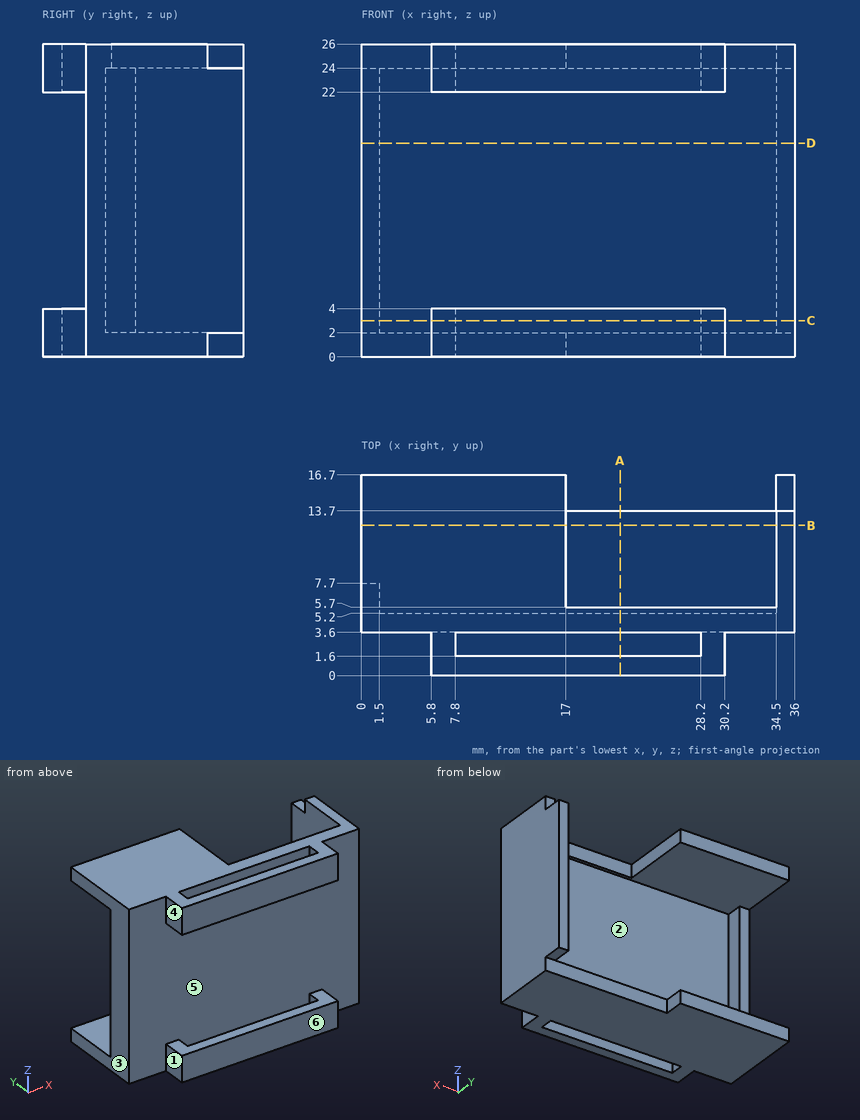
Can you work these out from the drawing? Everything is in mm from the part's minimum corner. A direction names the side the tool comes from. Give positions to 0.01 mm unless a question says otherwise; leave off trailing zeros. Write each loop counter-clockwise with the first axis right and the second up, starting at its lowest first coordinate (ties: lowest second). Pieces come first, ordered by that corner, then holes. Notation, with made-up numbers: (-4.5, 39) -> (40.5, 39) arc R30 ccw to (40.5, 68) -> close; hole circle Ø8 at (32, 30). An arc over 180 degrees is marked (long way). Write each question's results on one line, items separated by ' | '.
Item 1: If I drill on L1, parallel to Z at x = 15, y = 1; L2, parallel to Z at x = 28.5, y = 5.25; L3, parallel to X at y = 6.25, z = 3.5, over which ranges is the centre line in solid material (lowest first)?
Output:
L1: z = 0 to 4, 22 to 26 | L2: z = 0 to 2, 24 to 26 | L3: x = 0 to 1.5, 34.5 to 36
Item 2: Suppose I cut it at D-D on z = 17.75. Write out the boundary of the cut face in (x, y).
Output:
outline: (0, 3.6) -> (36, 3.6) -> (36, 16.7) -> (34.5, 16.7) -> (34.5, 5.2) -> (1.5, 5.2) -> (1.5, 7.7) -> (0, 7.7) -> close
Item 3: For pin 1 Ø1.1 at (y, z) = (1, 24) entering from -X; pin 2 Ø1.2 at (x, y) = (35.5, 15) entering from -Z; pin 3 Ø1.1 at (y, z) = (2, 24) entering from +X, each with a flat end and sliding along its axis, tell me the tip position at first contact or that it passes through.
Output:
pin 1: stops at x = 5.8 | pin 2: stops at z = 2 | pin 3: stops at x = 30.2
Item 4: We'd pull the mould along X, two halves only. Please class the marked faces 4, 5 and 6: pulls with the +X half, pulls with the -X half, needs draft (parallel to the pull), parting line crosses it, or undercut.
Output:
face 4: pulls with the -X half | face 5: undercut | face 6: needs draft
Item 5: Suppose I cut it at B-B on y = 12.5. Write out the boundary of the cut face in (x, z), plus the area to 3 significant figures.
Output:
outline: (0, 0) -> (36, 0) -> (36, 26) -> (34.5, 26) -> (34.5, 2) -> (0, 2) -> close; (0, 24) -> (17, 24) -> (17, 26) -> (0, 26) -> close | area: 142 mm^2
Item 6: On a 3-axis mill with a long thin cutter (end or side, diameter ignored), from which of +Z, -Z, +X, -X, +Y, -Y can I reach the whole of each face in a straight line? I mean the marked faces 1, 2 and 3. Say none if no direction works.
Output:
face 1: +Z, -Z, -X, -Y | face 2: +Y | face 3: +Z, -Z, -X, +Y, -Y
Item 7: Suppose I cut it at C-C on z = 3. Write out the boundary of the cut face in (x, y).
Output:
outline: (0, 3.6) -> (5.8, 3.6) -> (5.8, 0) -> (30.2, 0) -> (30.2, 3.6) -> (36, 3.6) -> (36, 16.7) -> (34.5, 16.7) -> (34.5, 5.2) -> (1.5, 5.2) -> (1.5, 7.7) -> (0, 7.7) -> close; hole (7.8, 1.6) -> (28.2, 1.6) -> (28.2, 3.6) -> (7.8, 3.6) -> close
Item 8: Suppose I cut it at A-A on x = 21.5. Write out the boundary of the cut face in (y, z).
Output:
outline: (0, 0) -> (1.6, 0) -> (1.6, 4) -> (0, 4) -> close; (0, 22) -> (1.6, 22) -> (1.6, 26) -> (0, 26) -> close; (3.6, 0) -> (13.7, 0) -> (13.7, 2) -> (5.2, 2) -> (5.2, 24) -> (5.7, 24) -> (5.7, 26) -> (3.6, 26) -> close
